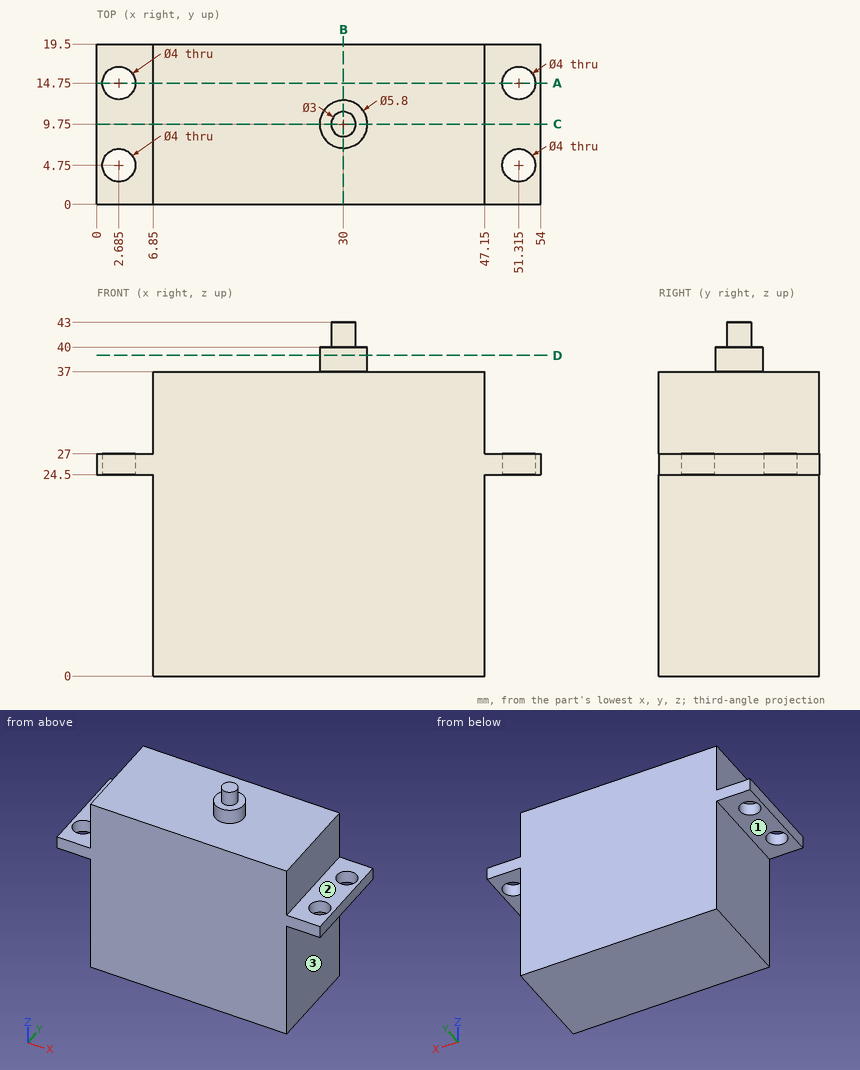
Geometry: see drawing. Coordinates: mm, zero at the bounding-box minimum. A direction names the side the tool comes from. Round coordinates to 2 decimals unless told otherwise and drop trailing zeros. Write each loop counter-clockwise with the first axis right and the second up, starting at its lowest first coordinate (ties: lowest second). Pieces come first, ordered by that corner, then holes. Notation, with made-up numbers: M 83,78 L 129,78 A21 cw 129,99 Z; hole C 88.5,21 d7. An arc over 180 degrees is marked long. Answer in a Markdown table with one row per item. Add a question column.
(1) Contact query for flat-ended pins moving along their axis: pin 1 (4 mm diameter, centred on x = 47, y = 2.5, fed in from +Z); pin 2 (2.5 mm diameter, centred on x = 2.685, y = 4.75, fed in from +Z); pin 3 (8 mm diameter, centred on y = 10, z = 38.5, fed in from +X); pin 4 (2 mm diameter, centred on y = 7.5, z = 30.5, fed in from -X). Output: stop coordinate, or through.
(2) Reachability of the marked faces 1, 2 and 3 from +Z, -Z, +X, -X, +Y, -Y: full face, straight path, thin tool, end or side. Return the list, or none.
(3) Cut plane A-A, the plane y = 14.75. Return the cut outline in (x, z) (3 decimals), then the cut area to 3 significant figures.
(4) Cut plane D-D, the plane z = 39. Return the cut outline in (x, y).
(5) Ray query, L1, parallel to Z at x = 9, y = 7; L2, parallel to X at y = 12.75, z = 18.5. Return the intervals inside material, ascending.
(6) Cut plane C-C, the plane y = 9.75. Return the cut outline in (x, z).
(7) Cut plane B-B, the plane x = 30. Return the cut outline in (y, z), then the cut area to 3 significant figures.
Established:
| question | item | result |
|---|---|---|
| 1 | pin 1 | z = 37 |
| 1 | pin 2 | through |
| 1 | pin 3 | x = 47.15 |
| 1 | pin 4 | x = 6.85 |
| 2 | face 1 | -Z, -X, +Y, -Y |
| 2 | face 2 | +Z, +X, +Y, -Y |
| 2 | face 3 | -Z, +X, +Y, -Y |
| 3 | outline | M 0,24.5 L 0.685,24.5 L 0.685,27 L 0,27 Z; M 4.685,24.5 L 6.85,24.5 L 6.85,0 L 47.15,0 L 47.15,24.5 L 49.315,24.5 L 49.315,27 L 47.15,27 L 47.15,37 L 6.85,37 L 6.85,27 L 4.685,27 Z; M 53.315,24.5 L 54,24.5 L 54,27 L 53.315,27 Z |
| 3 | area | 1,510 mm² |
| 4 | outline | C 30,9.75 d5.8 |
| 5 | L1 | 0 to 37 |
| 5 | L2 | 6.85 to 47.15 |
| 6 | outline | M 0,24.5 L 6.85,24.5 L 6.85,0 L 47.15,0 L 47.15,24.5 L 54,24.5 L 54,27 L 47.15,27 L 47.15,37 L 32.9,37 L 32.9,40 L 31.5,40 L 31.5,43 L 28.5,43 L 28.5,40 L 27.1,40 L 27.1,37 L 6.85,37 L 6.85,27 L 0,27 Z |
| 7 | outline | M 0,0 L 19.5,0 L 19.5,37 L 12.65,37 L 12.65,40 L 11.25,40 L 11.25,43 L 8.25,43 L 8.25,40 L 6.85,40 L 6.85,37 L 0,37 Z |
| 7 | area | 748 mm² |
